Input: part model. Units: mm. Frame: model coordinates. Face numbers are marked on the shaded views. Coordinates: 2 decimals unless noted, no trailing zeros. Order: outer loops, then holes, each group sorted by start corner. A loop starts at its lowest first (then second) coordinate and runs counter-clockwise, first axis right, second up. Notation, with made-up numbers: (42, -1) -> (71, -1) arc R13 cw to (71, 3) -> close; hole circle Ø6 at (85.5, -13.75). An arc over 180 degrees is marked (long way). One line per question, with ' | ' between items.
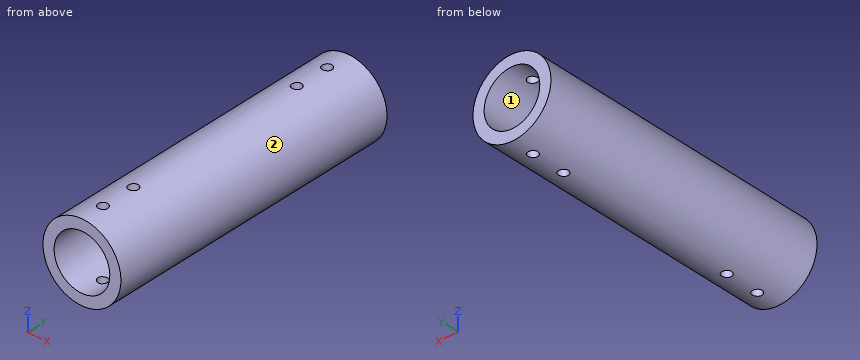
```python
from build123d import *

# Parameters (mm, degrees)
SKETCH1_R           = 13.335
SKETCH1_R_2         = 9.525
BOSS_EXTRUDE1_DEPTH = 105
SKETCH4_R           = 1.7
CUT_EXTRUDE1_DEPTH  = 107.680103346


with BuildPart() as part:
    # Sketch1 → Boss-Extrude1 (new body)
    with BuildSketch(Plane(origin=(0, 0, 0), x_dir=(1, 0, 0), z_dir=(0, 1, 0))):
        with Locations(Location((0, 0, 0), (0, 0, 270))):
            Circle(SKETCH1_R)
        with Locations(Location((0, 0, 0), (0, 0, 270))):
            Circle(SKETCH1_R_2, mode=Mode.SUBTRACT)
    extrude(amount=BOSS_EXTRUDE1_DEPTH)

    # Sketch4 → Cut-Extrude1 (cut, symmetric)
    with BuildSketch(Plane.XY):
        with Locations((0, 96.744231704)):
            Circle(SKETCH4_R)
        with Locations((0, 84.744231704)):
            Circle(SKETCH4_R)
    cut_extrude1 = extrude(amount=CUT_EXTRUDE1_DEPTH, both=True, mode=Mode.SUBTRACT)

    # Mirror2: Cut-Extrude1 across plane
    add(cut_extrude1.mirror(Plane.ZX.offset(52.5)), mode=Mode.SUBTRACT)


solid = part.part
```
1. Cut plane D-D, the plane y = 48.5. Return loops of the section in (x, z) (3 decimals), and give its area (3 significant figures).
Recorded:
outline: circle Ø26.67 at (0, 0); hole circle Ø19.05 at (0, 0) | area: 274 mm^2
2. Cut plane B-B, the plane z = -11.25. Return loops of the section in (x, y), and give its area (3 significant figures).
Recorded:
outline: (-7.16, 0) -> (7.16, 0) -> (7.16, 105) -> (-7.16, 105) -> close; hole circle Ø3.4 at (0, 8.26); hole circle Ø3.4 at (0, 20.26); hole circle Ø3.4 at (0, 84.74); hole circle Ø3.4 at (0, 96.74) | area: 1,470 mm^2
3. Pin query (flat end, axial travel): pin 1 Ø2.5 at (x, y) = (0, 8.26) entering from +Z; pin 2 Ø4 at (x, y) = (0, 96.74) entering from -Z (3 decimals); pin 3 Ø8 at (x, y) = (6, 80.5) entering from +Z; pin 4 Ø5 at (y, z) = (76.5, -6.5) entering from -X. Return the tip coordinate at first contact, or that it passes through.
Recorded:
pin 1: passes through | pin 2: stops at z = -13.335 | pin 3: stops at z = 13.18 | pin 4: stops at x = -12.72
4. Cut plane C-C, the plane x = 0. State how many separate pieces and enclosed holes the cut face has, and give its area (3 significant figures).
Recorded:
separate pieces: 10 | enclosed holes: 0 | area: 696 mm^2
5. Cut plane A-A, the plane z = -5. Return loops of the section in (x, y).
Recorded:
outline: (-12.36, 0) -> (-8.11, 0) -> (-8.11, 105) -> (-12.36, 105) -> close; (8.11, 0) -> (12.36, 0) -> (12.36, 105) -> (8.11, 105) -> close
6. Ray query, line 1 (X direction, y = 14.5, z = 0) (3 decimals); line 2 (Z direction, x = -0.25, y = 15.5); line 3 (Z direction, x = -4, y = 8). Return the intervals inside material, ascending. Write a range as [from, to].
Recorded:
line 1: x = [-13.335, -9.525], [9.525, 13.335] | line 2: z = [-13.33, -9.52], [9.52, 13.33] | line 3: z = [-12.72, -8.64], [8.64, 12.72]
7. Mould query, pull axis Z, two halves, no side actions, for the marked faces 1 and 2. Classes: released by +Z, released by -Z, zero draft, split by the parting line, or undercut.
Recorded:
face 1: undercut | face 2: split by the parting line
